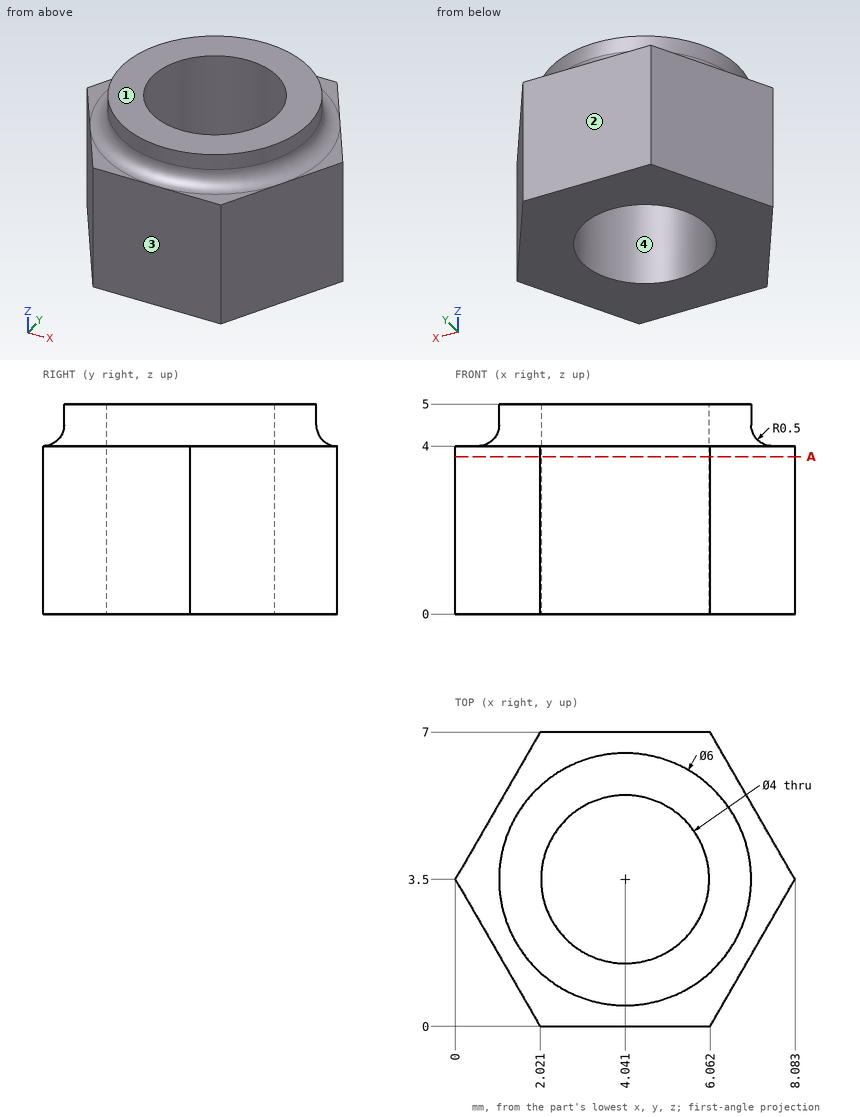
The figure shows three views and two pictorial views of one solid part (mm, origin at its lowest corner). Answer the questions. Round coordinates to 2 decimals unless told otherwise and drop trailing zeros. Order: outer loops, then holes, each group sorted by start corner. A loop starts at its lowest first (then second) coordinate and runs counter-clockwise, first axis right, second up. Notation, with made-up numbers: (-3.75, 65) - (25.25, 65) arc R22 ccw to (25.25, 84) - close; hole circle Ø2 at (18, -23). An arc over 180 degrees is marked (long way). Write item = value, one per line. Start each with the question number.
1) Section A-A, the plane z = 3.75 is taken. Write down the section's boundary in (x, y).
2) For a pull along Y with two mould halves and no side action, classify the marked faces 1, 2, 3 and 4 as released by +Y, released by -Y, zero draft, split by the parting line, or undercut.
3) Given pin 1 (3 mm diameter, centred on x = 4, y = 3.5, fed in from -Z); pin 2 (3.5 mm diameter, centred on x = 4.5, y = 2.5, fed in from +Z); pin 3 (3 mm diameter, centred on y = 6, z = 3.5, fed in from +X) (1 decimal); pin 4 (1 mm diameter, centred on x = 7, y = 1, fed in from +Z), each flat-ended and moving along its own axis, determine where each tip first touches the part or whether it passes through.
4) Straight lines are drawn through the part: L1, parallel to Y at x = 4, z = 3.85; L2, parallel to Y at x = 5.5, z = 4.3; L3, parallel to X at y = 5, z = 2.35 (1 decimal). For each, find the intervals that lie inside material, in ascending order.
Results list:
q1.outline = (0, 3.5) - (2.02, 0) - (6.06, 0) - (8.08, 3.5) - (6.06, 7) - (2.02, 7) - close; hole circle Ø4 at (4.04, 3.5)
q2.face_1 = zero draft
q2.face_2 = released by +Y
q2.face_3 = released by -Y
q2.face_4 = undercut
q3.pin_1 = through
q3.pin_2 = 5
q3.pin_3 = 7.5
q3.pin_4 = 4.02
q4.L1 = 0 to 1.5, 5.5 to 7
q4.L2 = 0.83 to 2.13, 4.87 to 6.17
q4.L3 = 0.9 to 2.7, 5.4 to 7.2
